Could you check a few things on this model? Use its own coordinates, in mm. A direction names the side the tool comes from. Give positions to 0.01 mm unless a question says otherwise; leave off trailing zeros. Order: outer loops, then holes, each group sorted by start corner. A loop starts at its lowest first (then second) coordinate and runs counter-clockwise, first axis right, second up. Notation, with made-up numbers: M -9,9.25 L 44,9.25 A31 cw 44,35.25 Z; hole C -38.75,-40 d10. An arc over 180 degrees is marked long. Use a Markdown table: item, result. Add a question column.
Item 1: Suppose I cut it at B-B on y = 3.1. Write out the boundary of the cut face in (x, z) (3 decimals).
Item 2: Suppose I cut it at C-C on z = 2. Write out the boundary of the cut face in (x, y).
Item 3: For faces 1 (the face through (0, 2, -6)), 2 (the face through (-2.588, 3.718, 1.467)), which set-ups out of +Z, -Z, +X, -X, +Y, -Y let a thin tool reach every point of the face, with its end or its side?
Item 4: Suppose I cut it at A-A on z = -0.25. Write out the boundary of the cut face in (x, y).
Item 5: Suppose I cut it at D-D on y = 0.6. Write out the boundary of the cut face in (x, z), plus the area to 3 significant figures.
Item 6: If we mould it in two halves opening along Y, with no side actions, what happens to faces 3 (the face through (1.5, 2.4, -0.7)), 4 (the face through (1.2, 0, -1.4)), 5 (the face through (0, 4, 2.975))? For each: released by +Y, released by -Y, zero draft, split by the parting line, or undercut.
Item 7: If I drill on L1, parallel to X at y = 1.6, z = 0; L2, parallel to Z at x = 0.5, y = 2.85 (3 decimals); L3, parallel to X at y = 4.75, z = -0.25, over which ranges is the centre line in solid material (lowest first)? Write a range as from..to.
from build123d import *

# Parameters (mm, degrees)
SKETCH1_W           = 12
SKETCH1_H           = 12
BOSS_EXTRUDE1_DEPTH = 5
SKETCH2_R           = 1.5
CUT_EXTRUDE1_DEPTH  = 5
CUT_EXTRUDE2_DEPTH  = 2.6


with BuildPart() as part:
    # Sketch1 → Boss-Extrude1 (new body)
    with BuildSketch(Plane(origin=(0, 0, 0), x_dir=(1, 0, 0), z_dir=(0, 1, 0))):
        Rectangle(SKETCH1_W, SKETCH1_H)
    extrude(amount=BOSS_EXTRUDE1_DEPTH)

    # Sketch2 → Cut-Extrude1 (cut)
    with BuildSketch(Plane(origin=(0, 5, 0), x_dir=(1, 0, 0), z_dir=(0, 1, 0))):
        with Locations(Location((0, 0, 0), (0, 0, 270))):
            Circle(SKETCH2_R)
    extrude(amount=-CUT_EXTRUDE1_DEPTH, mode=Mode.SUBTRACT)

    # Sketch3 → Cut-Extrude2 (cut)
    with BuildSketch(Plane(origin=(0, 5, 0), x_dir=(1, 0, 0), z_dir=(0, 1, 0))):
        Polygon((3.435234102, 0), (1.717617051, 2.975), (-1.717617051, 2.975), (-3.435234102, 0), (-1.717617051, -2.975), (1.717617051, -2.975), align=None)
    extrude(amount=-CUT_EXTRUDE2_DEPTH, mode=Mode.SUBTRACT)


solid = part.part
Findings below:
| question | item | result |
|---|---|---|
| 1 | outline | M -6,-6 L 6,-6 L 6,6 L -6,6 Z; hole M -3.435,0 L -1.718,-2.975 L 1.718,-2.975 L 3.435,0 L 1.718,2.975 L -1.718,2.975 Z |
| 2 | outline | M -6,0 L 6,0 L 6,5 L 2.28,5 L 2.28,2.4 L -2.28,2.4 L -2.28,5 L -6,5 Z |
| 3 | face 1 | -Z, +X, -X, +Y, -Y |
| 3 | face 2 | +Y |
| 4 | outline | M -6,0 L -1.48,0 L -1.48,2.4 L -3.29,2.4 L -3.29,5 L -6,5 Z; M 1.48,0 L 6,0 L 6,5 L 3.29,5 L 3.29,2.4 L 1.48,2.4 Z |
| 5 | outline | M -6,-6 L 6,-6 L 6,6 L -6,6 Z; hole C 0,0 d3 |
| 5 | area | 137 mm^2 |
| 6 | face 3 | released by +Y |
| 6 | face 4 | released by -Y |
| 6 | face 5 | zero draft |
| 7 | L1 | x = -6..-1.5, 1.5..6 |
| 7 | L2 | z = -6..-2.975, 2.975..6 |
| 7 | L3 | x = -6..-3.29, 3.29..6 |
